Read the model definition and answer for the solid it produces. Units are mm, in the model's axes. Face numbers are marked on the shaded views. A direction names the side the tool comes from. Round coordinates to 2 decimals unless told otherwise and drop trailing zeros. Order: outer loops, then holes, each group sorted by start corner. A loop starts at its lowest first (then second) coordinate and runs counter-clockwise, first axis right, second up. Notation, with made-up numbers: (48.25, 49) - (60.25, 49) arc R19 cw to (60.25, 55) - close; hole circle Ø4 at (59, 79.25). An arc over 180 degrees is marked (long way). Put each result on its own line as item: value. Start each with the question number.
Q1. Section C-C on y = -18 is taken. Give the vertices of the cut face in (x, z).
Q2. Each of these flat-tipped pins is pushed along its axis until it touches: pin 1 Ø1 at (x, z) = (-29.5, 86) entering from -Y; pin 2 Ø2 at (y, z) = (-4, 49) entering from -X; pin 3 Ø5 at (y, z) = (43, 29) entering from -X. Where does it stop, or does it pass through?
Q3. For a pull along Y with two mould halves and no side action, classify the marked faces 3, 4 and 5 as pulls with the +Y half, pulls with the -Y half, needs draft (parallel to the pull), parting line crosses it, or undercut.
Q4. Section B-B on x = -9.5 is taken. Give the vertices of the cut face in (y, z).
Q5. Find the intervals of material crossed by line 1 along Y through (x, z) = (2, 92.5); line 2 along X through (y, z) = (23, 28.5); line 3 along Y through (x, z) = (36, 26.5), in increasing order. Write a range as from..to.
Q6. Section A-A on z = 71.5 is taken. Give the vertices of the cut face in (x, y), then the cut area to 3 significant figures.
Q7. Which of the six approach directions +Z, -Z, +X, -X, +Y, -Y give full straight-line access (tool end or side, diameter ignored) to the marked faces 1 and 2?
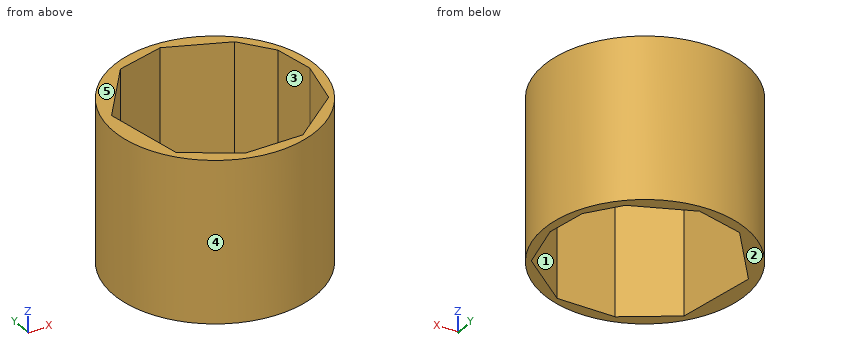
from build123d import *

# Parameters (mm, degrees)
F0_R     = 63.5
F1_DEPTH = 101.6
F2_DEPTH = 101.6
F3_DEPTH = 25.4
F4_DEPTH = 101.6


with BuildPart() as f1:
    # F0 (on Top) → F1 (new body)
    with BuildSketch(Plane.XY):
        Circle(F0_R)
        Polygon((-15.682541, -56.195769), (-46.46679, -36.447387), (-56.050561, 13.50441), (-27.299238, 51.549092), (2.032924, 59.099946), (38.915936, 43.707822), (54.017641, 24.540273), (58.954742, 0), (51.984716, -30.639039), (20.32922, -56.195769), align=None, mode=Mode.SUBTRACT)
    extrude(amount=F1_DEPTH)

    # F0 (on Top) → F2 (join)
    with BuildSketch(Plane.XY):
        Circle(F0_R)
        Polygon((-15.682541, -56.195769), (-46.46679, -36.447387), (-56.050561, 13.50441), (-27.299238, 51.549092), (2.032924, 59.099946), (38.915936, 43.707822), (54.017641, 24.540273), (58.954742, 0), (51.984716, -30.639039), (20.32922, -56.195769), align=None, mode=Mode.SUBTRACT)
    extrude(amount=F2_DEPTH)

    # F0 (on Top) → F3 (join)
    with BuildSketch(Plane.XY):
        Circle(F0_R)
        Polygon((-15.682541, -56.195769), (-46.46679, -36.447387), (-56.050561, 13.50441), (-27.299238, 51.549092), (2.032924, 59.099946), (38.915936, 43.707822), (54.017641, 24.540273), (58.954742, 0), (51.984716, -30.639039), (20.32922, -56.195769), align=None, mode=Mode.SUBTRACT)
    extrude(amount=F3_DEPTH)

    # F0 (on Top) → F4 (join)
    with BuildSketch(Plane.XY):
        Circle(F0_R)
        Polygon((-15.682541, -56.195769), (-46.46679, -36.447387), (-56.050561, 13.50441), (-27.299238, 51.549092), (2.032924, 59.099946), (38.915936, 43.707822), (54.017641, 24.540273), (58.954742, 0), (51.984716, -30.639039), (20.32922, -56.195769), align=None, mode=Mode.SUBTRACT)
    extrude(amount=F4_DEPTH)


solid = f1.part
Findings:
1. outline: (-60.9, 0) - (-50.01, 0) - (-50.01, 101.6) - (-60.9, 101.6) - close; (54.86, 0) - (60.9, 0) - (60.9, 101.6) - (54.86, 101.6) - close
2. pin 1: y = -56.49
2. pin 2: x = -63.43
2. pin 3: x = -48.91
3. face 3: undercut
3. face 4: parting line crosses it
3. face 5: needs draft
4. outline: (-62.79, 0) - (-56.2, 0) - (-56.2, 101.6) - (-62.79, 101.6) - close; (56.13, 0) - (62.79, 0) - (62.79, 101.6) - (56.13, 101.6) - close
5. line 1: -63.47..-56.2, 59.09..63.47
5. line 2: -59.19..-48.87, 54.33..59.19
5. line 3: -52.31..-43.54, 44.92..52.31
6. outline: circle Ø127 at (0, 0); hole (-56.05, 13.5) - (-46.47, -36.45) - (-15.68, -56.2) - (20.33, -56.2) - (51.98, -30.64) - (58.95, 0) - (54.02, 24.54) - (38.92, 43.71) - (2.03, 59.1) - (-27.3, 51.55) - close
6. area: 2,600 mm2
7. face 1: +Z, -Z
7. face 2: -Z, +X, -X, +Y, -Y
